Here's how the part is built. I have some questions about the finished solid (model axes, mm). Face numbers are marked on the shaded views. A direction names the side the tool comes from. Give positions to 0.01 mm unless a question says otherwise; leave off trailing zeros. Write each loop counter-clockwise with the first axis right and the second up, starting at its lowest first coordinate (ties: lowest second). Pieces come first, ordered by that corner, then holes. Notation, with made-up numbers: (-24, 15) - (-7, 15) arc R8 cw to (-7, 19) - close; hole circle Ø5 at (-18.5, 36.25). An arc over 180 degrees is marked (long way). One line per item, written item: value. Start each with the question number.
1) Imagine slicing it at A-A on y = 3. Write out the boundary of the cut face in (x, z).
2) Imagine slicing it at D-D on y = -5. Write out the boundary of the cut face in (x, z).
3) On a 3-axis mill with a long thin cutter (end or side, diameter ignored), from which of +Z, -Z, +X, -X, +Y, -Y can I reach the whole of each face in a straight line? I mean the marked faces 1 and 2. Say none if no direction works.
4) Imagine slicing it at B-B on z = 0. Write out the boundary of the cut face in (x, y).
5) Please list where these lines run through material, in increasing order: L1, parallel to Z at x = 15.5, y = 2.2; L2, parallel to Z at x = -15, y = 2. Write a range as [from, to].
6) Imagine slicing it at C-C on x = 0. Write out the boundary of the cut face in (y, z).
7) I'm going to push flat-ended pins straight in: P1, Ø3, axis at x = -14, y = -3, coming from the -Z side; P2, Ø3, axis at x = -15.5, z = -15.5, coming from the -Y side; P3, Ø3.5, axis at x = 0.5, y = -10, coming from the -Z side. Where does each tip first touch, or does it pass through?
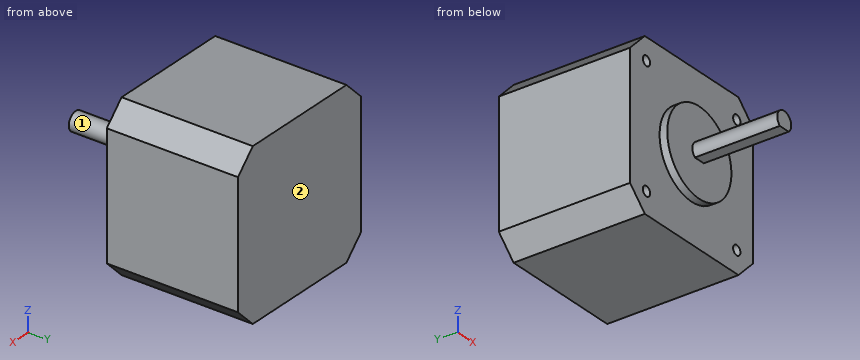
from build123d import *

# Parameters (mm, degrees)
BOSS_EXTRUDE1_DEPTH       = 34
M3X0_5_TAPPED_HOLE1_D     = 2.5
M3X0_5_TAPPED_HOLE1_DEPTH = 4.499991
M3X0_5_TAPPED_HOLE1_TIP   = 0.751075774
SKETCH4_R                 = 11
BOSS_EXTRUDE2_DEPTH       = 2
BOSS_EXTRUDE3_DEPTH       = 22


with BuildPart() as part:
    # Sketch1 → Boss-Extrude1 (new body)
    with BuildSketch(Plane(origin=(0, 0, 0), x_dir=(1, 0, 0), z_dir=(0, 1, 0))):
        Polygon((-21.15, -16.07), (-21.15, 16.07), (-16.07, 21.15), (16.07, 21.15), (21.15, 16.07), (21.15, -16.07), (16.07, -21.15), (-16.07, -21.15), align=None)
    extrude(amount=BOSS_EXTRUDE1_DEPTH)

    # M3x0.5 Tapped Hole1
    with Locations(Plane(origin=(0, 0, 0), x_dir=(-1, 0, 0), z_dir=(0, -1, 0))):
        with Locations((-15.5, 15.5), (15.5, 15.5), (15.5, -15.5), (-15.5, -15.5)):
            Hole(M3X0_5_TAPPED_HOLE1_D / 2, depth=M3X0_5_TAPPED_HOLE1_DEPTH)
            with Locations((0, 0, -(M3X0_5_TAPPED_HOLE1_DEPTH + M3X0_5_TAPPED_HOLE1_TIP / 2))):  # 118° drill point
                Cone(0, M3X0_5_TAPPED_HOLE1_D / 2, M3X0_5_TAPPED_HOLE1_TIP, mode=Mode.SUBTRACT)

    # Sketch4 → Boss-Extrude2 (add)
    with BuildSketch(Plane(origin=(0, 0, 0), x_dir=(-1, 0, 0), z_dir=(0, -1, 0))):
        Circle(SKETCH4_R)
    extrude(amount=BOSS_EXTRUDE2_DEPTH)

    # Sketch5 → Boss-Extrude3 (add)
    with BuildSketch(Plane.XZ.offset(2)):
        with BuildLine():
            Line((1.524, -1.848854431), (-1.524, -1.848854431))
            ThreePointArc((-1.524, -1.848854431), (0, 2.396004738), (1.524, -1.848854431))
        make_face()
    extrude(amount=BOSS_EXTRUDE3_DEPTH)


solid = part.part
Numbers:
1. outline: (-21.15, -16.07) - (-16.07, -21.15) - (16.07, -21.15) - (21.15, -16.07) - (21.15, 16.07) - (16.07, 21.15) - (-16.07, 21.15) - (-21.15, 16.07) - close; hole circle Ø2.5 at (-15.5, -15.5); hole circle Ø2.5 at (-15.5, 15.5); hole circle Ø2.5 at (15.5, -15.5); hole circle Ø2.5 at (15.5, 15.5)
2. outline: (-1.52, -1.85) - (1.52, -1.85) arc R2.4 ccw (long way) to start
3. face 1: -Y
3. face 2: +Z, -Z, +X, -X, +Y
4. outline: (-21.15, 0) - (-11, 0) - (-11, -2) - (-2.4, -2) - (-2.4, -24) - (2.4, -24) - (2.4, -2) - (11, -2) - (11, 0) - (21.15, 0) - (21.15, 34) - (-21.15, 34) - close
5. L1: [-21.15, -16.75], [-14.25, 14.25], [16.75, 21.15]
5. L2: [-21.15, -16.65], [-14.35, 14.35], [16.65, 21.15]
6. outline: (-24, -1.85) - (-2, -1.85) - (-2, -11) - (0, -11) - (0, -21.15) - (34, -21.15) - (34, 21.15) - (0, 21.15) - (0, 11) - (-2, 11) - (-2, 2.4) - (-24, 2.4) - close
7. P1: through
7. P2: y = 0
7. P3: z = -1.85
